Verification items for the finished model (mm, model axes). A direction names the side the tool comes from. Round coordinates to 2 decimals unless told otherwise and drop trailing zeros. Order: outer loops, then holes, each group sorted by start corner. A loop starts at its lowest first (then second) coordinate and runs counter-clockwise, first axis right, second up. Notation, with made-up numbers: M 69,-12.5 L 111,-12.5 A25 cw 111,16.5 Z; hole C 55,68.25 d5. An arc over 180 degrees is marked long. Use one line per item in the form item = value. Start each with the question number.
Item 1: Cross-section at D-D on x = 15. Enter the section's corners in (y, z).
Item 2: Cross-section at C-C on y = 16. Enter the section's corners in (x, z), then the cut area to 3 significant figures.
Item 3: Tool access check on faces 1 (the flat face through (-12.5, -23, 2)), 2 (the cylindrical face through (10.59, 25.19, 3.07)), 3 (the flat face through (12.5, 18, 2)). Record the directions out of +Z, -Z, +X, -X, +Y, -Y that give a thin tool (end or side, any length) a straight path to the whole face; none if there is none.
Item 4: Thickness scan on probe 1 along Y at (x, z) = (0, 2.15); probe 2 along Y at (x, z) = (0, 2.7); probe 3 along X at (y, z) = (23.5, 2.5). Record the ranges inside material, lowest first. Write a range as [from, to].
Item 5: Go/stop test with flat-tipped pins: pin 1 Ø3 at (x, y) = (-6.7, -11.7) entering from +Z; pin 2 Ø2 at (x, z) = (-9.5, 2.5) entering from -Y; pin 3 Ø1 at (y, z) = (11, 2) entering from -X; pin 4 Ø2 at (x, z) = (9.5, 2.5) entering from +Y. Record where each tip stops, or that it passes through.
Item 6: Cross-section at B-B on y = -27. Enter the section's corners in (x, z), then the cut area to 3 significant figures.
Item 7: Cross-section at A-A on x = 0. Enter the section's corners in (y, z).
Item 8: Release check for a two-part mould opening along Y. For faces 4 (the cylindrical face through (-3, 3.4, 2.2)), 5 (the cylindrical face through (10.59, -25.19, 1.93)), 6 (the cylindrical face through (6.5, -28.2, 2.5)) record: +Y half, -Y half, draft (parallel to the pull), parting line (faces both ways), or undercut.
Autodesk Inventor part; units mm, degrees
ref_plane "YZ Plane" through (0, 0, 0) normal (1, 0, 0) x (0, 1, 0)
ref_plane "XZ Plane" through (0, 0, 0) normal (0, 1, 0) x (-1, 0, 0)
ref_plane "XY Plane" through (0, 0, 0) normal (0, 0, 1) x (1, 0, 0)
sketch "スケッチ1" plane through (0, 0, 0) normal (0, 0, 1) x (1, 0, 0)
  line L0 (-12.5, 29.25) -> (12.5, 29.25)
  line L1 (12.5, 29.25) -> (12.5, -29.25)
  line L2 (12.5, -29.25) -> (-12.5, -29.25)
  line L3 (-12.5, -29.25) -> (-12.5, 29.25)
  line L4 (-12.5, 29.25) -> (12.5, -29.25) construction
  line L5 (12.5, 29.25) -> (-12.5, -29.25) construction
  line L6 (-5.5, 29.25) -> (-5.5, 31.25)
  line L7 (-5.5, 31.25) -> (5.5, 31.25)
  line L8 (0, 29.25) -> (0, -29.25) construction
  line L9 (5.5, 29.25) -> (5.5, 31.25)
  arc A0 (-7.6, 29.25) -> (-5.5, 29.25) centre (-6.55, 29.25) ccw
  arc A1 (5.5, 29.25) -> (7.6, 29.25) centre (6.55, 29.25) ccw
  line L10 (-12.5, 0) -> (12.5, 0) construction
  line L11 (-5.5, -29.25) -> (-5.5, -31.25)
  line L12 (-5.5, -31.25) -> (5.5, -31.25)
  line L13 (5.5, -29.25) -> (5.5, -31.25)
  arc A2 (-5.5, -29.25) -> (-7.6, -29.25) centre (-6.55, -29.25) ccw
  arc A3 (7.6, -29.25) -> (5.5, -29.25) centre (6.55, -29.25) ccw
  circle A4 centre (0, -5) radius 13.95 construction
  circle A5 centre (0, -5) radius 14.05
  circle A6 centre (-6.6998, -11.6998) radius 1.55
  line L14 (-9.9349, -14.9349) -> (0, -5) construction
  circle A7 centre (6.6998, -11.6998) radius 1.55
  circle A8 centre (6.6998, 1.6998) radius 1.55
  circle A9 centre (-6.6998, 1.6998) radius 1.55
  circle A10 centre (0, -5) radius 4
  circle A11 centre (0, -13.5) radius 3
  circle A12 centre (8.5, -5) radius 3
  circle A13 centre (0, 3.5) radius 3
  circle A14 centre (-8.5, -5) radius 3
  arc A15 (-10.6051, 8.3504) -> (-12.5, -16.5954) centre (0, -5) ccw
  arc A16 (12.5, -16.5954) -> (10.6051, 8.3504) centre (0, -5) ccw
  point P0 (0, 0)
  point P1 (-5.5, -29.25)
  point P2 (5.5, -29.25)
  point P3 (7.6, 29.25)
  point P4 (5.5, -29.25)
  point P5 (-5.5, -29.25)
  point P6 (-12.5, 1.415)
  point P7 (12.5, 1.415)
  point P8 (12.5, -11.415)
  point P9 (-12.5, -11.415)
  point P10 (12.5, -16.5954)
  point P11 (12.5, 6.5954)
  point P12 (-12.5, 6.5954)
  dimension "d0" = 25
  dimension "d1" = 58.5
  dimension "d2" = 11
  dimension "d3" = 2
  dimension "d4" = 1.05
  dimension "d13" = 27.9
  dimension "d17" = 24.25
  dimension "d44" = 0.1
  dimension "d48" = 3.1
  dimension "d49" = 45
  dimension "d50" = 9.475
  dimension "d53" = 360
  dimension "d55" = 8
  dimension "d56" = 6
  dimension "d57" = 8.5
  dimension "d60" = 360
  dimension "d64" = 3
extrude "押し出し1" add sketch "スケッチ1" along normal blind 5 contours L0 A0 A1 L1 A5 L3 | L3 A5 A15 | L3 A5 L1 L2 A3 A2 | L1 A16 A5
extrude "押し出し2" add sketch "スケッチ1" along normal blind 2.5 contours L6 L7 L9 L0 | L2 L13 L12 L11
sketch "スケッチ2" plane through (-12.5, -29.25, 0) normal (0, -1, 0) x (1, 0, 0)
  line L0 (0, 0) -> (4.9, 0)
  line L1 (12.5, 5) -> (12.5, 0) construction
  line L2 (0, 0) -> (25, 0)
  line L3 (0, 5) -> (25, 5)
  point P0 (3, 2.5)
  point P1 (22, 2.5)
  point P2 (20.1, 0)
  point P3 (7, 5)
  point P4 (18, 5)
  point P5 (7, 0)
  dimension "d26" = 2.5
  dimension "d27" = 19
hole "穴1" at (-9.5, -29.25, 2.5) at (9.5, -29.25, 2.5) direction (0, 1, 0) diameter 2.459 depth 8 tip angle 118
sketch "スケッチ3" plane through (-12.5, 29.25, 0) normal (0, 1, 0) x (1, 0, 0)
  circle A0 centre (22, -2.5) radius 1.2295
  circle A1 centre (3, -2.5) radius 1.2295
  point P0 (12.5, 0)
hole "穴2" at (9.5, 29.25, 2.5) at (-9.5, 29.25, 2.5) direction (0, -1, 0) diameter 2.459 depth 8 tip angle 118
extrude "押し出し3" add sketch "スケッチ1" along normal blind 4.5 contours A5 L1 L3 | L3 A5 | A5 L1
fillet "フィレット3" radius 2 4 edges at (-12.5, -16.5954, 2.5) (-12.5, 6.5954, 2.5) (12.5, 6.5954, 2.5) (12.5, -16.5954, 2.5)
properties part number "Leg_joint_basis_frame" material "アルミニウム 2014-T4"
Output values:
q1.outline = M -13.11,0 L 3.11,0 L 3.11,5 L -13.11,5 Z
q2.outline = M -12.5,0 L 12.5,0 L 12.5,5 L -12.5,5 Z
q2.area = 125 mm2
q3.face_1 = +Z, -Z, -X, -Y
q3.face_2 = +Y
q3.face_3 = +Z, -Z, +X, +Y
q4.probe_1 = [-31.25, -16.5], [-10.5, -9], [-1, 0.5], [6.5, 31.25]
q4.probe_2 = [-29.25, -16.5], [-10.5, -9], [-1, 0.5], [6.5, 29.25]
q4.probe_3 = [-12.5, -10.73], [-8.27, 8.27], [10.73, 12.5]
q5.pin_1 = through
q5.pin_2 = -21.11
q5.pin_3 = -12.5
q5.pin_4 = 21.11
q6.outline = M -12.5,0 L 12.5,0 L 12.5,5 L -12.5,5 Z; hole C -9.5,2.5 d2.46; hole C 9.5,2.5 d2.46
q6.area = 116 mm2
q7.outline = M -31.25,0 L -16.5,0 L -16.5,4.5 L -19.05,4.5 L -19.05,5 L -29.25,5 L -29.25,2.5 L -31.25,2.5 Z; M -10.5,0 L -9,0 L -9,4.5 L -10.5,4.5 Z; M -1,0 L 0.5,0 L 0.5,4.5 L -1,4.5 Z; M 6.5,0 L 31.25,0 L 31.25,2.5 L 29.25,2.5 L 29.25,5 L 9.05,5 L 9.05,4.5 L 6.5,4.5 Z
q8.face_4 = undercut
q8.face_5 = draft
q8.face_6 = -Y half
